Can you work these out from the model? Positions are in its coordinate system, mm. Face numbers are marked on the shaded views. A direction names the side the tool comes from. Give positions to 0.01 mm unless a question says otherwise; leave off trailing zeros. Loops run counter-clockwise (first coordinate to the right, second up) from the corner with the lowest first, then second, coordinate; pieces in that order, holes last. Notation, with made-up numbers: (59.5, -3.5) - (64.5, -3.5) arc R30 cw to (64.5, 35.5) - close; hole circle Ø1 at (68.25, 9.25). An arc over 180 degrees is marked (long way). Answer as a JSON object with one key per item and string values.
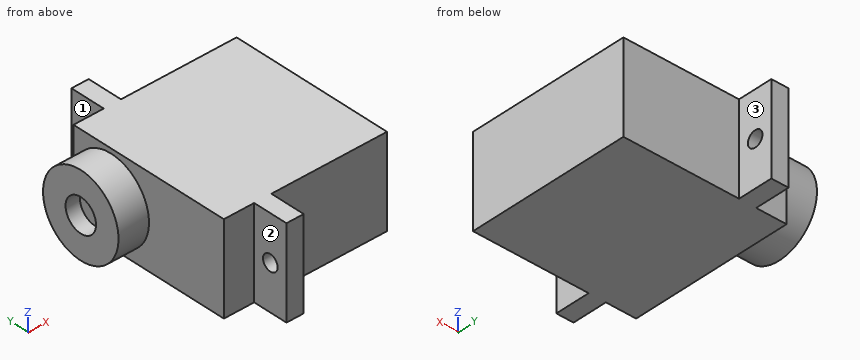
```python
from build123d import *

# Parameters (mm, degrees)
SKETCH1_W           = 22.75
SKETCH1_H           = 22.7
BOSS_EXTRUDE1_DEPTH = 12.5
SKETCH2_R           = 5.7
BOSS_EXTRUDE2_DEPTH = 4.25
SKETCH3_R           = 2.3
CUT_EXTRUDE1_DEPTH  = 2
SKETCH4_W           = 12.5
SKETCH4_H           = 4.875
BOSS_EXTRUDE3_DEPTH = 2.4
SKETCH5_R           = 1.1
CUT_EXTRUDE2_DEPTH  = 2.4


with BuildPart() as part:
    # Sketch1 → Boss-Extrude1 (new body)
    with BuildSketch(Plane.XY):
        Rectangle(SKETCH1_W, SKETCH1_H)
    extrude(amount=BOSS_EXTRUDE1_DEPTH)

    # Sketch2 → Boss-Extrude2 (add)
    with BuildSketch(Plane.ZY.offset(11.375)):
        with Locations(Location((6.152972547, 5.65, 0), (0, 0, 90))):
            Circle(SKETCH2_R)
    extrude(amount=BOSS_EXTRUDE2_DEPTH)

    # Sketch3 → Cut-Extrude1 (cut)
    with BuildSketch(Plane.ZY.offset(15.625)):
        with Locations((6.152972547, 5.65)):
            Circle(SKETCH3_R)
    extrude(amount=-CUT_EXTRUDE1_DEPTH, mode=Mode.SUBTRACT)

    # Sketch4 → Boss-Extrude3 (add)
    with BuildSketch(Plane(origin=(-7.15, 0, 0), x_dir=(0, 0, -1), z_dir=(1, 0, 0))):
        with Locations((-6.25, 13.7875)):
            Rectangle(SKETCH4_W, SKETCH4_H)
        with Locations((-6.25, -13.7875)):
            Rectangle(SKETCH4_W, SKETCH4_H)
    extrude(amount=BOSS_EXTRUDE3_DEPTH)

    # Sketch5 → Cut-Extrude2 (cut)
    with BuildSketch(Plane.ZY.offset(7.15)):
        with Locations((6.25, 13.7875)):
            Circle(SKETCH5_R)
        with Locations(Location((6.25, -13.7875, 0), (0, 0, 180))):
            Circle(SKETCH5_R)
    extrude(amount=-CUT_EXTRUDE2_DEPTH, mode=Mode.SUBTRACT)


solid = part.part
```
1) I'm going to push flat-ended pins straight in: P1, Ø1.3, axis at x = -10, z = 9, coming from the +Y side; P2, Ø1.3, axis at x = -8.5, z = 3.5, coming from the -Y side; P3, Ø5.5, axis at y = 14, z = 8.5, coming from the -X side (3 decimals); P4, Ø2, axis at y = 13.79, z = 6.25, coming from the +X side. Where does each tip first touch, or does it pass through?
Check sheet entries:
{"P1": "y = 11.35", "P2": "y = -11.35", "P3": "x = -11.375", "P4": "through"}
2) Imagine slicing it at D-D on x = 7. Write out the boundary of the cut face in (y, z), and give its area (3 significant figures).
Check sheet entries:
{"outline": "(-11.35, 0) - (11.35, 0) - (11.35, 12.5) - (-11.35, 12.5) - close", "area": "284 mm2"}
3) Imagine slicing it at C-C on x = -6.75. Give the number of separate pieces and of enclosed holes in the cut face, and give its area (3 significant figures).
Check sheet entries:
{"separate pieces": "1", "enclosed holes": "2", "area": "398 mm2"}
4) I need wall thicknesses on L1, parallel to Y at x = -6.35, z = 6.25 (1 decimal); L2, parallel to Y at x = -5.5, z = 6.75 (3 decimals); L3, parallel to X at y = -9, z = 10.5 (3 decimals). Which ranges of each line are inside material? Lowest first, please.
Check sheet entries:
{"L1": "-16.2 to -14.9, -12.7 to 12.7, 14.9 to 16.2", "L2": "-16.225 to -14.767, -12.808 to 12.808, 14.767 to 16.225", "L3": "-11.375 to 11.375"}
5) Imagine slicing it at A-A on z = 5.75. Write out the boundary of the cut face in (x, y) (3 decimals).
Check sheet entries:
{"outline": "(-15.625, -0.036) - (-11.375, -0.036) - (-11.375, -11.35) - (-7.15, -11.35) - (-7.15, -12.808) - (-4.75, -12.808) - (-4.75, -11.35) - (11.375, -11.35) - (11.375, 11.35) - (-4.75, 11.35) - (-4.75, 12.808) - (-7.15, 12.808) - (-7.15, 11.35) - (-11.375, 11.35) - (-11.375, 11.336) - (-15.625, 11.336) - (-15.625, 7.914) - (-13.625, 7.914) - (-13.625, 3.386) - (-15.625, 3.386) - close; (-7.15, -16.225) - (-4.75, -16.225) - (-4.75, -14.767) - (-7.15, -14.767) - close; (-7.15, 14.767) - (-4.75, 14.767) - (-4.75, 16.225) - (-7.15, 16.225) - close"}
6) Which directions (+Z, -Z, +X, -X, +Y, -Y) give clear straight access to the entire face, cutting with the end or side of a thin tool? Please do the marked faces 1, 2 and 3.
Check sheet entries:
{"face 1": "+Z, -Z, -X, +Y", "face 2": "+Z, -Z, -X, -Y", "face 3": "+Z, -Z, +X, +Y"}
7) Imagine slicing it at B-B on y = 5.65. Write out the boundary of the cut face in (x, z) (3 decimals).
Check sheet entries:
{"outline": "(-15.625, 0.453) - (-11.375, 0.453) - (-11.375, 0) - (11.375, 0) - (11.375, 12.5) - (-11.375, 12.5) - (-11.375, 11.853) - (-15.625, 11.853) - (-15.625, 8.453) - (-13.625, 8.453) - (-13.625, 3.853) - (-15.625, 3.853) - close"}
